from build123d import *

# Parameters (mm, degrees)
BOSS_EXTRUDE1_DEPTH     = 431.8
SKETCH2_W               = 136.525
SKETCH2_H               = 4.7625
CUT_EXTRUDE1_DEPTH      = 455.272910918
SKETCH3_W               = 132.265960651
SKETCH3_H               = 13.462
CUT_EXTRUDE2_DEPTH      = 455.272910918
SKETCH4_W               = 11.600566843
SKETCH4_H               = 14.103653616
SKETCH4_W_2             = 12.2809
SKETCH4_H_2             = 14.918520238
CUT_EXTRUDE3_DEPTH      = 454.414011969
CUT_EXTRUDE4_DEPTH      = 454.047023636
CUT_EXTRUDE4_DEPTH_BACK = 454.047023636
SKETCH5_W               = 16.6878
SKETCH5_H               = 17.155999978
SKETCH5_W_2             = 119.8372
FILLET1_R               = 2.54
M6_CLEARANCE_HOLE2_D    = 6.6


with BuildPart() as part:
    # Sketch1 → Boss-Extrude1 (new body)
    with BuildSketch(Plane(origin=(0, 0, 0), x_dir=(1, 0, 0), z_dir=(0, 1, 0))):
        with BuildLine():
            Line((0, 0), (136.525, 0))
            Line((136.525, 0), (136.525, 9.525))
            Line((136.525, 9.525), (132.5372, 9.525))
            Line((132.5372, 9.525), (132.5372, 34.925))
            ThreePointArc((132.5372, 34.925), (131.7752, 35.687), (131.0132, 34.925))
            Line((131.0132, 34.925), (131.0132, 9.525))
            Line((131.0132, 9.525), (126.1872, 9.525))
            Line((126.1872, 9.525), (126.1872, 34.925))
            ThreePointArc((126.1872, 34.925), (125.4252, 35.687), (124.6632, 34.925))
            Line((124.6632, 34.925), (124.6632, 9.525))
            Line((124.6632, 9.525), (119.8372, 9.525))
            Line((119.8372, 9.525), (119.8372, 34.925))
            ThreePointArc((119.8372, 34.925), (119.0752, 35.687), (118.3132, 34.925))
            Line((118.3132, 34.925), (118.3132, 9.525))
            Line((118.3132, 9.525), (113.4872, 9.525))
            Line((113.4872, 9.525), (113.4872, 34.925))
            ThreePointArc((113.4872, 34.925), (112.7252, 35.687), (111.9632, 34.925))
            Line((111.9632, 34.925), (111.9632, 9.525))
            Line((111.9632, 9.525), (107.1372, 9.525))
            Line((107.1372, 9.525), (107.1372, 34.925))
            ThreePointArc((107.1372, 34.925), (106.3752, 35.687), (105.6132, 34.925))
            Line((105.6132, 34.925), (105.6132, 9.525))
            Line((105.6132, 9.525), (100.7872, 9.525))
            Line((100.7872, 9.525), (100.7872, 34.925))
            ThreePointArc((100.7872, 34.925), (100.0252, 35.687), (99.2632, 34.925))
            Line((99.2632, 34.925), (99.2632, 9.525))
            Line((99.2632, 9.525), (94.4372, 9.525))
            Line((94.4372, 9.525), (94.4372, 34.925))
            ThreePointArc((94.4372, 34.925), (93.6752, 35.687), (92.9132, 34.925))
            Line((92.9132, 34.925), (92.9132, 9.525))
            Line((92.9132, 9.525), (88.0872, 9.525))
            Line((88.0872, 9.525), (88.0872, 34.925))
            ThreePointArc((88.0872, 34.925), (87.3252, 35.687), (86.5632, 34.925))
            Line((86.5632, 34.925), (86.5632, 9.525))
            Line((86.5632, 9.525), (81.7372, 9.525))
            Line((81.7372, 9.525), (81.7372, 34.925))
            ThreePointArc((81.7372, 34.925), (80.9752, 35.687), (80.2132, 34.925))
            Line((80.2132, 34.925), (80.2132, 9.525))
            Line((80.2132, 9.525), (75.3872, 9.525))
            Line((75.3872, 9.525), (75.3872, 34.925))
            ThreePointArc((75.3872, 34.925), (74.6252, 35.687), (73.8632, 34.925))
            Line((73.8632, 34.925), (73.8632, 9.525))
            Line((73.8632, 9.525), (69.0372, 9.525))
            Line((69.0372, 9.525), (69.0372, 34.925))
            ThreePointArc((69.0372, 34.925), (68.2752, 35.687), (67.5132, 34.925))
            Line((67.5132, 34.925), (67.5132, 9.525))
            Line((67.5132, 9.525), (62.6872, 9.525))
            Line((62.6872, 9.525), (62.6872, 34.925))
            ThreePointArc((62.6872, 34.925), (61.9252, 35.687), (61.1632, 34.925))
            Line((61.1632, 34.925), (61.1632, 9.525))
            Line((61.1632, 9.525), (56.3372, 9.525))
            Line((56.3372, 9.525), (56.3372, 34.925))
            ThreePointArc((56.3372, 34.925), (55.5752, 35.687), (54.8132, 34.925))
            Line((54.8132, 34.925), (54.8132, 9.525))
            Line((54.8132, 9.525), (49.9872, 9.525))
            Line((49.9872, 9.525), (49.9872, 34.925))
            ThreePointArc((49.9872, 34.925), (49.2252, 35.687), (48.4632, 34.925))
            Line((48.4632, 34.925), (48.4632, 9.525))
            Line((48.4632, 9.525), (43.6372, 9.525))
            Line((43.6372, 9.525), (43.6372, 34.925))
            ThreePointArc((43.6372, 34.925), (42.8752, 35.687), (42.1132, 34.925))
            Line((42.1132, 34.925), (42.1132, 9.525))
            Line((42.1132, 9.525), (37.2872, 9.525))
            Line((37.2872, 9.525), (37.2872, 34.925))
            ThreePointArc((37.2872, 34.925), (36.5252, 35.687), (35.7632, 34.925))
            Line((35.7632, 34.925), (35.7632, 9.525))
            Line((35.7632, 9.525), (30.9372, 9.525))
            Line((30.9372, 9.525), (30.9372, 34.925))
            ThreePointArc((30.9372, 34.925), (30.1752, 35.687), (29.4132, 34.925))
            Line((29.4132, 34.925), (29.4132, 9.525))
            Line((29.4132, 9.525), (24.5872, 9.525))
            Line((24.5872, 9.525), (24.5872, 34.925))
            ThreePointArc((24.5872, 34.925), (23.8252, 35.687), (23.0632, 34.925))
            Line((23.0632, 34.925), (23.0632, 9.525))
            Line((23.0632, 9.525), (18.2372, 9.525))
            Line((18.2372, 9.525), (18.2372, 34.925))
            ThreePointArc((18.2372, 34.925), (17.4752, 35.687), (16.7132, 34.925))
            Line((16.7132, 34.925), (16.7132, 9.525))
            Line((16.7132, 9.525), (11.8872, 9.525))
            Line((11.8872, 9.525), (11.8872, 34.925))
            ThreePointArc((11.8872, 34.925), (11.1252, 35.687), (10.3632, 34.925))
            Line((10.3632, 34.925), (10.3632, 9.525))
            Line((10.3632, 9.525), (5.5372, 9.525))
            Line((5.5372, 9.525), (5.5372, 34.925))
            ThreePointArc((5.5372, 34.925), (4.7752, 35.687), (4.0132, 34.925))
            Line((4.0132, 34.925), (4.0132, 9.525))
            Line((4.0132, 9.525), (0, 9.525))
            Line((0, 9.525), (0, 0))
        make_face()
    extrude(amount=BOSS_EXTRUDE1_DEPTH)

    # Sketch2 → Cut-Extrude1 (cut, through all)
    with BuildSketch(Plane(origin=(0, 431.8, 0), x_dir=(1, 0, 0), z_dir=(0, 1, 0))):
        with Locations((68.2625, 2.38125)):
            Rectangle(SKETCH2_W, SKETCH2_H)
    extrude(amount=-CUT_EXTRUDE1_DEPTH, mode=Mode.SUBTRACT)

    # Sketch3 → Cut-Extrude2 (cut, through all)
    with BuildSketch(Plane.XZ):
        with Locations((69.2831702, -28.956)):
            Rectangle(SKETCH3_W, SKETCH3_H)
    extrude(amount=-CUT_EXTRUDE2_DEPTH, mode=Mode.SUBTRACT)

    # Sketch4 → Cut-Extrude3 (cut, through all)
    with BuildSketch(Plane(origin=(0, 431.8, 0), x_dir=(1, 0, 0), z_dir=(0, 1, 0))):
        with Locations((7.806883422, 16.576826808)):
            Rectangle(SKETCH4_W, SKETCH4_H)
        with Locations((128.39065, 16.984260119)):
            Rectangle(SKETCH4_W_2, SKETCH4_H_2)
    extrude(amount=-CUT_EXTRUDE3_DEPTH, mode=Mode.SUBTRACT)

    # Sketch5 → Cut-Extrude4 (cut, two sides: drawn at the far end of the back side and taken through both)
    with BuildSketch(Plane(origin=(0, 0, -9.525), x_dir=(-1, 0, 0), z_dir=(0, 0, -1)).offset(-CUT_EXTRUDE4_DEPTH_BACK)):
        with Locations((-128.1811, 8.577999989)):
            Rectangle(SKETCH5_W, SKETCH5_H)
        with Locations((-59.9186, 8.577999989)):
            Rectangle(SKETCH5_W_2, SKETCH5_H)
    extrude(amount=CUT_EXTRUDE4_DEPTH + CUT_EXTRUDE4_DEPTH_BACK, mode=Mode.SUBTRACT)

    # Fillet1
    fillet1_edges = [part.edges().sort_by_distance(p)[0] for p in [
        (136.525, 431.8, -7.14375),
        (0, 431.8, -7.14375),
        (0, 17.155999978, -7.14375),
        (136.525, 17.155999978, -7.14375),
    ]]
    fillet(fillet1_edges, radius=FILLET1_R)

    # M6 Clearance Hole2 (through all)
    with Locations(Plane.XY.offset(-4.7625)):
        with Locations((9.324759355, 31.310999989), (129.902965514, 31.310999989), (130.630936095, 110.558999989), (9.324759355, 100.652999989), (9.324759355, 179.900999989), (130.630936095, 189.806999989), (9.324759355, 259.148999989), (130.630936095, 269.054999989), (130.630936095, 348.302999989), (9.324759355, 338.396999989), (9.324759355, 417.644999989), (129.902965514, 417.644999989)):
            Hole(M6_CLEARANCE_HOLE2_D / 2)


solid = part.part
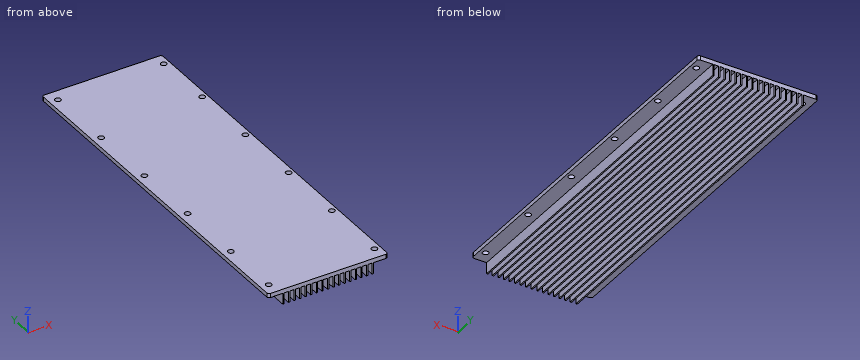
Design review of the part built by this model. Coordinates are the model's own, in mm. Give positions to 0.01 mm unless a question says otherwise; leave off trailing zeros. Write item = value, one per line.
1) Clearance check with flat-ended pins moving along their axes: pin 1 Ø2 at (y, z) = (137.5, -15) entering from -X; pin 2 Ø1.4 at (x, y) = (91, 253.5) entering from -Z (3 decimals); pin 3 Ø6 at (x, y) = (9.32, 259.15) entering from +Z; pin 4 Ø1 at (y, z) = (112.5, -14.5) entering from +X. State where each tip first meets the part, or that it passes through.
Result sheet:
pin_1 = 16.71
pin_2 = -9.525
pin_3 = through
pin_4 = 119.84
2) Take a section at A-A on z = -12.75. Count the separate pieces of the cut face and the enclosed holes in it, and give its area (3 significant figures).
Result sheet:
separate_pieces = 17
enclosed_holes = 0
area = 10,700 mm2
3) To check wall thickness, follow line 1 (Z direction, x = 41, y = 362.5) (1 decimal). State the ranges of the line that lie inside material, in increasing order.
Result sheet:
line_1 = -9.5 to -4.8
